The listing builds one solid part. Answer for the finished solid, in the listing's coordinates (mm). A direction names the side the tool comes from. Coordinates: 2 decimals unless noted, no trailing zeros. Order: outer loops, then holes, each group sorted by start corner. A loop starts at its lowest first (then second) coordinate and runs counter-clockwise, first axis right, second up.
from build123d import *

# Parameters (mm, degrees)
F0_R     = 3.5
F1_DEPTH = 1.5
F2_R     = 3
F3_DEPTH = 8
F4_R     = 2
F5_DEPTH = 7.7
F6_R     = 2.429154
F7_DEPTH = 0.5


with BuildPart() as f1:
    # F0 (on Front) → F1 (new body)
    with BuildSketch(Plane.XZ):
        with Locations((-14.26011, 19.491863)):
            Circle(F0_R)
    extrude(amount=F1_DEPTH)

    # F2 (on face) → F3 (join)
    with BuildSketch(Plane.XZ.offset(1.5)):
        with Locations((-14.26011, 19.491863)):
            Circle(F2_R)
    extrude(amount=F3_DEPTH)

    # F4 (on face) → F5 (join)
    with BuildSketch(Plane.XZ.offset(9.5)):
        with Locations((-14.26011, 19.491863)):
            Circle(F4_R)
    extrude(amount=F5_DEPTH)

    # F6 (on face) → F7 (cut)
    with BuildSketch(Plane(origin=(0, 0, 0), x_dir=(-1, 0, 0), z_dir=(0, 1, 0))):
        with Locations((14.26011, 19.491863)):
            Circle(F6_R)
    extrude(amount=-F7_DEPTH, mode=Mode.SUBTRACT)


solid = f1.part
1) Section A-A (x = -12) is taken. Give the vertices of the cut face in (y, z).
2) Section D-D (x = -15.75) is taken. Give the vertices of the cut face in (y, z).
3) Determine the mould class of faces 4 (the face through (-14, -0.5, 20)), 5 (the face through (-14, -17.2, 20)), 6 (the face through (-17.757, -0.74, 19.646)) for opening direction X: released by +X, released by -X, zero draft, split by the parting line, or undercut.
4) Each of these flat-tipped pins is pushed along its axis until it touches: P1, Ø2.5, axis at x = -13.5, z = 20, coming from the +Y side; P2, Ø3, axis at y = -12.5, z = 17.5, coming from the -X side; P3, Ø4, axis at x = -16.5, y = -8, coming from the +Z side; P4, Ø4, axis at x = -16.5, z = 18, coming from the +Y side. Where does it stop, or does it pass through?
5) A tool of negligible diameter and unlimited length cuts with its end or side. For faces 1 (the face through (-15.566, -0.246, 21.54)), 2 (the face through (-15, 0, 17)), 3 (the face through (-13.185, -13.296, 21.178)), from which of +Z, -Z, +X, -X, +Y, -Y can it reach the whole face along a straight path? Write none if from no direction.
6) Section C-C (y = -8.5) is taken. Give the vertices of the cut face in (x, z), then the cut area to 3 significant figures.
7) Consider L1, parallel to X at y = -7.5, z = 19.5; L2, parallel to Z at x = -16.5, y = -2.5; L3, parallel to Z at x = -14.25, y = -8.5. Determine where each line is inside the solid, lowest interval first.
8) Section B-B (z = 22.25) is taken. Give the vertices of the cut face in (x, y), then the cut area to 3 significant figures.
Filled sheet:
1. outline: (-9.5, 17.52) - (-1.5, 17.52) - (-1.5, 16.82) - (0, 16.82) - (0, 18.6) - (-0.5, 18.6) - (-0.5, 20.38) - (0, 20.38) - (0, 22.16) - (-1.5, 22.16) - (-1.5, 21.46) - (-9.5, 21.46) - close
2. outline: (-17.2, 18.16) - (-9.5, 18.16) - (-9.5, 16.89) - (-1.5, 16.89) - (-1.5, 16.32) - (0, 16.32) - (0, 17.57) - (-0.5, 17.57) - (-0.5, 21.41) - (0, 21.41) - (0, 22.66) - (-1.5, 22.66) - (-1.5, 22.1) - (-9.5, 22.1) - (-9.5, 20.83) - (-17.2, 20.83) - close
3. face 4: undercut
3. face 5: zero draft
3. face 6: split by the parting line
4. P1: stops at y = -0.5
4. P2: stops at x = -16.2
4. P3: stops at z = 22.48
4. P4: stops at y = 0
5. face 1: +Y
5. face 2: +Z, -Z, +X, -X, +Y
5. face 3: -Y
6. outline: circle Ø6 at (-14.26, 19.49)
6. area: 28.3 mm2
7. L1: x = -17.26 to -11.26
7. L2: z = 17.5 to 21.49
7. L3: z = 16.49 to 22.49
8. outline: (-16.41, -1.5) - (-15.44, -1.5) - (-15.44, -9.5) - (-13.08, -9.5) - (-13.08, -1.5) - (-12.11, -1.5) - (-12.11, 0) - (-16.41, 0) - close
8. area: 25.3 mm2
